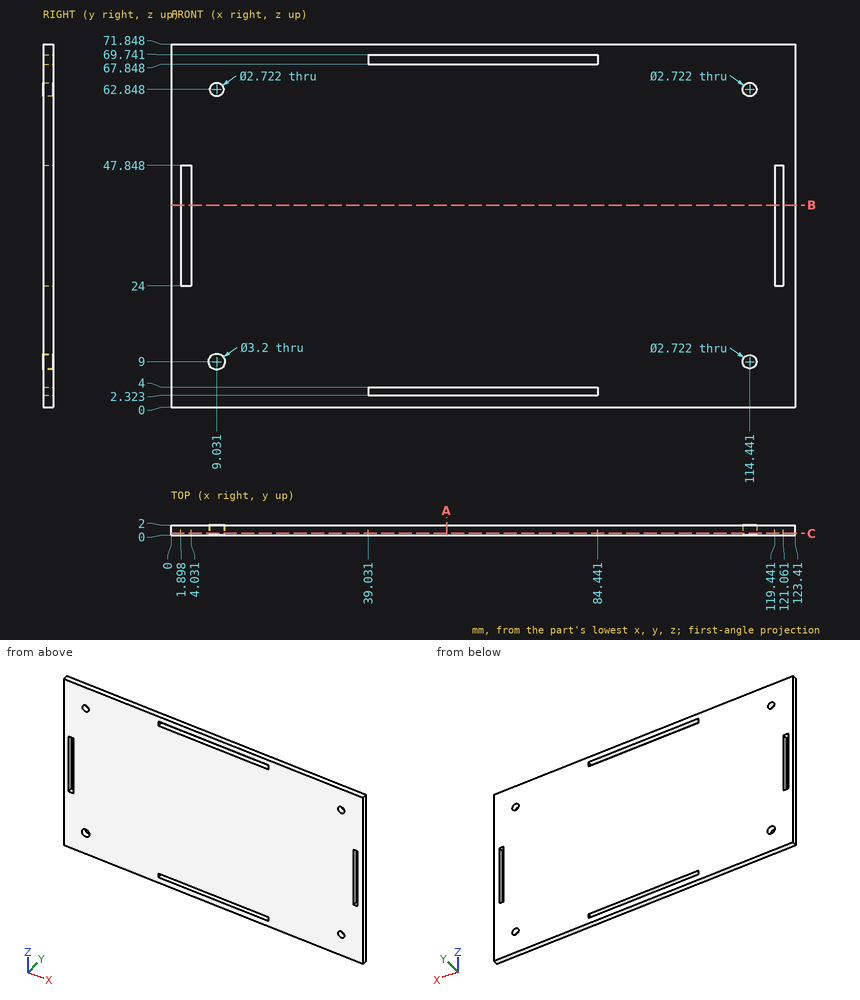
Answer from the drawing. Dimensions are ordinates in mm from the lowest x, y and z of the part. Give positions to 0.01 mm unless a question says otherwise; leave off trailing zeros. Order: outer loops, then holes, each group sorted by start corner. A loop starts at its lowest first (then second) coordinate and runs counter-clockwise, first axis right, second up. Notation, with made-up numbers: (-3.5, 46) -> (31.5, 46) arc R30 cw to (31.5, 82) -> close; hole circle Ø9 at (-21.5, 55.25). An arc over 180 degrees is marked (long way). One line per item, written item: value.
Item 1: Find section A-A, the plane x = 54.5. Give the vertices of the cut face in (y, z).
Answer sheet:
outline: (0, 0) -> (2, 0) -> (2, 2.32) -> (0, 2.32) -> close; (0, 4) -> (2, 4) -> (2, 67.85) -> (0, 67.85) -> close; (0, 69.74) -> (2, 69.74) -> (2, 71.85) -> (0, 71.85) -> close
Item 2: Find section B-B, the plane z = 40. Give the vertices of the cut face in (x, y).
Answer sheet:
outline: (0, 0) -> (1.9, 0) -> (1.9, 2) -> (0, 2) -> close; (4.03, 0) -> (119.44, 0) -> (119.44, 2) -> (4.03, 2) -> close; (121.06, 0) -> (123.41, 0) -> (123.41, 2) -> (121.06, 2) -> close
Item 3: Straight lines are drawn through the part: probe 1 along X at (y, z) = (1.2, 34); probe 2 along X at (y, z) = (1, 9); probe 3 along Z at (x, y) = (68, 1.65). For each, find the intervals that lie inside material, in ascending order.
Answer sheet:
probe 1: 0 to 1.9, 4.03 to 119.44, 121.06 to 123.41
probe 2: 0 to 7.43, 10.63 to 113.08, 115.8 to 123.41
probe 3: 0 to 2.32, 4 to 67.85, 69.74 to 71.85
Item 4: Find section C-C, the plane y = 0.4. State how many separate pieces and enclosed holes the cut face has, plus the area to 3 significant figures.
Answer sheet:
separate pieces: 1
enclosed holes: 8
area: 8,590 mm²
